from build123d import *

# Parameters (mm, degrees)
F0_R        = 6
F1_DEPTH    = 10
F2_T1_DEPTH = 10
F3_W        = 40
F3_H        = 52
F4_DEPTH    = 10
F5_R        = 8


# Not quite as in the source:
# - a fillet or chamfer that OpenCascade refuses, or shapes differently, is made with other operations: its cross-section is extruded or revolved along the edge and cut away or added


with BuildPart() as f1:
    # F0 (on Front) → F1 (new body)
    with BuildSketch(Plane.XZ):
        with BuildLine():
            Line((32, 52), (0, 52))
            Line((0, 52), (0, 0))
            Line((0, 0), (32, 0))
            Line((32, 0), (32, 13.0432075486))
            Line((32, 13.0432075486), (88, 13.0432075486))
            ThreePointArc((88, 13.0432075486), (102, 27.0432075486), (88, 41.0432075486))
            Line((88, 41.0432075486), (32, 41.0432075486))
            Line((32, 41.0432075486), (32, 52))
        make_face()
        with Locations((20, 12)):
            Circle(F0_R, mode=Mode.SUBTRACT)
        with Locations((20, 40)):
            Circle(F0_R, mode=Mode.SUBTRACT)
        with BuildLine():
            ThreePointArc((88, 33.0432075486), (94, 27.0432075486), (88, 21.0432075486))
            Line((88, 21.0432075486), (42.3112809658, 21.0432075486))
            ThreePointArc((42.3112809658, 21.0432075486), (36.3112809658, 27.0432075486), (42.3112809658, 33.0432075486))
            Line((42.3112809658, 33.0432075486), (88, 33.0432075486))
        make_face(mode=Mode.SUBTRACT)
    extrude(amount=F1_DEPTH)

    # F2: fillet of radius 12 on 2 edges, made by hand

    # F2_s2 → F2_t1 (join)
    with BuildSketch(Plane.XZ):
        with BuildLine():
            ThreePointArc((43.9545689178, 41.0432075486), (35.8465016568, 44.1967819828), (32, 52))
            Line((32, 52), (32, 41.0432075486))
            Line((32, 41.0432075486), (43.9545689178, 41.0432075486))
        make_face()
        with BuildLine():
            ThreePointArc((32, 1.0432075486), (35.5147186258, 9.5284889228), (44, 13.0432075486))
            Line((44, 13.0432075486), (32, 13.0432075486))
            Line((32, 13.0432075486), (32, 1.0432075486))
        make_face()
    extrude(amount=F2_T1_DEPTH)

    # F3 (on face) → F4 (join)
    with BuildSketch(Plane(origin=(0, 0, 0), x_dir=(0, -1, 0), z_dir=(-1, 0, 0))):
        with Locations((20, 26)):
            Rectangle(F3_W, F3_H)
        with BuildLine():
            ThreePointArc((33.1354735655, 11), (36.1354735655, 8), (33.1354735655, 5))
            Line((33.1354735655, 5), (24.4329432571, 5))
            ThreePointArc((24.4329432571, 5), (22.054313259, 8), (24.4329432571, 11))
            Line((24.4329432571, 11), (33.1354735655, 11))
        make_face(mode=Mode.SUBTRACT)
        with BuildLine():
            ThreePointArc((33.1354735655, 47), (36.1354735655, 44), (33.1354735655, 41))
            Line((33.1354735655, 41), (25.1354735655, 41))
            ThreePointArc((25.1354735655, 41), (22.1354735655, 44), (25.1354735655, 47))
            Line((25.1354735655, 47), (33.1354735655, 47))
        make_face(mode=Mode.SUBTRACT)
    extrude(amount=F4_DEPTH)

    # F5
    f5_edges = [f1.edges().sort_by_distance(p)[0] for p in [
        (-5, -40, 52),
        (-5, -40, 0),
    ]]
    fillet(f5_edges, radius=F5_R)


solid = f1.part
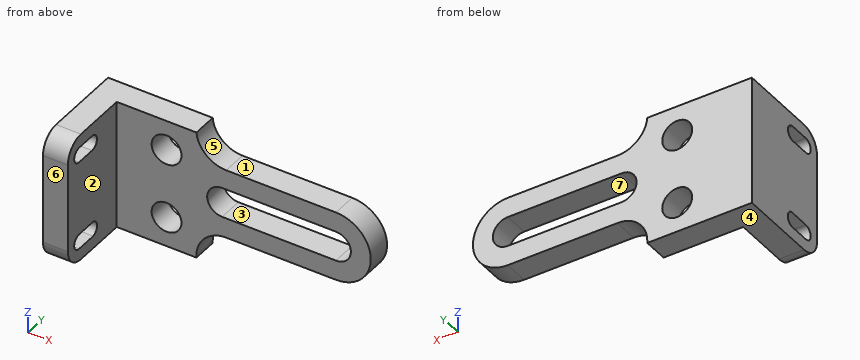
Here's how the part is built. I have some questions about the finished solid (model axes, mm). Face numbers are marked on the shaded views. A direction names the side the tool comes from. Coordinates: 2 decimals unless noted, no trailing zeros. Order: outer loops, then holes, each group sorted by start corner. A loop starts at its lowest first (then second) coordinate and runs counter-clockwise, first axis right, second up.
Item 1: If we section it at A-A on x = 20: List the corners of the cut face in (y, z) for me, plus the area to 3 significant figures.
Result sheet:
outline: (-10, 0) - (0, 0) - (0, 6) - (-10, 6) - close; (-10, 18) - (0, 18) - (0, 34) - (-10, 34) - close; (-10, 46) - (0, 46) - (0, 52) - (-10, 52) - close
area: 280 mm2
Item 2: I need wall thicknesses on line 1 (Z direction, x = 20, y = -3); line 2 (X direction, y = -21, z = 20). Which ranges of each line are inside material? Lowest first, please.
Result sheet:
line 1: z = 0 to 6, 18 to 34, 46 to 52
line 2: x = -10 to 0
Item 3: For the marked faces 1, 2 and 3, which set-ups out of +Z, -Z, +X, -X, +Y, -Y let a thin tool reach every point of the face, with its end or its side?
Result sheet:
face 1: +Z, +X, +Y, -Y
face 2: +Z, -Z, +X, -Y
face 3: +Y, -Y
Item 4: If we section it at D-D on x = 63: List the corners of the cut face in (y, z) for me.
Result sheet:
outline: (-10, 13.04) - (0, 13.04) - (0, 21.04) - (-10, 21.04) - close; (-10, 33.04) - (0, 33.04) - (0, 41.04) - (-10, 41.04) - close
Item 5: If we section it at B-B on y = -27: List the corners of the cut face in (x, z) for me.
Result sheet:
outline: (-10, 0) - (0, 0) - (0, 5) - (-10, 5) - close; (-10, 11) - (0, 11) - (0, 41) - (-10, 41) - close; (-10, 47) - (0, 47) - (0, 52) - (-10, 52) - close
Item 6: If we section it at C-C on z = 30: List the corners of the cut face in (x, y) for me.
Result sheet:
outline: (-10, -40) - (0, -40) - (0, -10) - (37.09, -10) - (37.09, 0) - (-10, 0) - close; (93.22, -10) - (101.68, -10) - (101.68, 0) - (93.22, 0) - close
Item 7: For P1, Ø14, axis at x = 20, z = 40, coming from the -Y side; P2, Ø4, axis at y = -17, z = 21, coming from the +X side; P3, Ø12, axis at x = 61.5, y = -14, coming from the -Z side; P4, Ø6, axis at x = 35.5, z = 40, coming from the +Y side, each with a flat end and sliding along its axis, tell me the tip position at first contact or that it passes through.
Result sheet:
P1: stops at y = -10
P2: stops at x = 0
P3: stops at z = 13.04
P4: stops at y = 0
Item 8: If we mould it in two halves opening along Z, with no side actions, what happens to the marked faces 4, 5, 6 and 7? For each: +Z half, -Z half, draft (parallel to the pull), parting line (faces both ways), or undercut.
Result sheet:
face 4: -Z half
face 5: +Z half
face 6: draft
face 7: undercut
